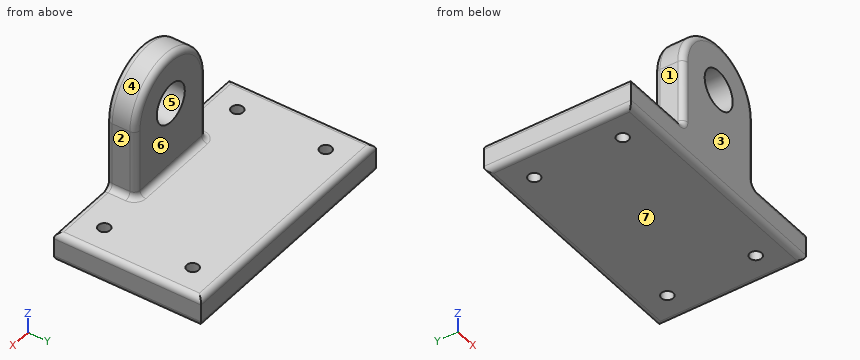
```python
from build123d import *

# Parameters (mm, degrees)
F0_W     = 125
F0_H     = 75
F1_DEPTH = 15
F2_W     = 50
F2_H     = 15
F3_DEPTH = 15
F4_R     = 3
F5_DEPTH = 15.001
F6_R     = 3


with BuildPart() as f1:
    # F0 (on Top) → F1 (new body)
    with BuildSketch(Plane.XY):
        Rectangle(F0_W, F0_H)
    extrude(amount=F1_DEPTH)

    # F2 (on face) → F3 (join)
    with BuildSketch(Plane.XZ.offset(37.5)):
        with Locations((0, 7.5)):
            Rectangle(F2_W, F2_H)
        with BuildLine():
            Line((25, 15), (25, 50))
            ThreePointArc((25, 50), (0, 25), (-25, 50))
            Line((-25, 50), (-25, 15))
            Line((-25, 15), (25, 15))
        make_face()
        with BuildLine():
            ThreePointArc((-25, 50), (0, 25), (25, 50))
            Line((25, 50), (10, 50))
            ThreePointArc((10, 50), (0, 40), (-10, 50))
            Line((-10, 50), (-25, 50))
        make_face()
        with BuildLine():
            Line((10, 50), (25, 50))
            ThreePointArc((25, 50), (0, 75), (-25, 50))
            Line((-25, 50), (-10, 50))
            ThreePointArc((-10, 50), (0, 60), (10, 50))
        make_face()
    extrude(amount=-F3_DEPTH)

    # F4 (on face) → F5 (cut, through all)
    with BuildSketch(Plane.XY.offset(15)):
        with Locations((-47.5, 22.5)):
            Circle(F4_R)
        with Locations((-47.5, -22.5)):
            Circle(F4_R)
        with Locations((47.5, 22.5)):
            Circle(F4_R)
        with Locations((47.5, -22.5)):
            Circle(F4_R)
    extrude(amount=-F5_DEPTH, mode=Mode.SUBTRACT)

    # F6
    f6_edges = [f1.edges().sort_by_distance(p)[0] for p in [
        (-43.75, -37.5, 15),
        (-62.5, 0, 15),
        (0, 37.5, 15),
        (62.5, 0, 15),
        (43.75, -37.5, 15),
        (25, -30, 15),
        (-25, -30, 15),
        (-25, -22.5, 32.5),
        (0, -37.5, 0),
        (62.5, 0, 0),
        (0, 37.5, 0),
        (-62.5, 0, 0),
        (-25, -37.5, 32.5),
        (0, -37.5, 75),
        (25, -37.5, 32.5),
        (0, -22.5, 15),
        (0, -22.5, 75),
        (25, -22.5, 32.5),
    ]]
    fillet(f6_edges, radius=F6_R)


solid = f1.part
```
Check sheet for the modelled part. Datum: model origin and axes. Units: mm. Face numbers are marked on the shaded views. A direction names the side the tool comes from. Give positions to 0.01 mm unless a question says otherwise; leave off trailing zeros. Order: outer loops, then holes, each group sorted by start corner. A loop starts at its lowest first (then second) coordinate and runs counter-clockwise, first axis right, second up. Notation, with made-up numbers: (0.25, 14.25) -> (55.25, 14.25) arc R18 ccw to (55.25, 48.25) -> close; hole circle Ø8 at (-14.5, 18.5). An arc over 180 degrees is marked (long way). Return JSON: item names as keys, results as strings.
1. Cross-section at C-C, the plane y = 22.5. Record the cut outline in (x, z), plus the area to 3 significant figures.
From the geometry:
{"outline": "(-62.5, 3) arc R3 ccw to (-59.5, 0) -> (-50.5, 0) -> (-50.5, 15) -> (-59.5, 15) arc R3 ccw to (-62.5, 12) -> close; (-44.5, 0) -> (44.5, 0) -> (44.5, 15) -> (-44.5, 15) -> close; (50.5, 0) -> (59.5, 0) arc R3 ccw to (62.5, 3) -> (62.5, 12) arc R3 ccw to (59.5, 15) -> (50.5, 15) -> close", "area": "1,690 mm^2"}
2. Set-up check for the marked faces 1, 2 and 3: record each of +Z, -Z, +X, -X, +Y, -Y from which the full face is reachable in a straight line by a thin tool's end or side.
From the geometry:
{"face 1": "+Z, -X, +Y, -Y", "face 2": "+Z, +X, +Y, -Y", "face 3": "+Z, -Z, +X, -X, -Y"}
3. Material ranges on probe 1 along Y at (x, z) = (-47.5, 4.5); probe 2 along Z at (x, y) = (0, -28); probe 3 along Z at (x, y) = (-33.5, 4.5), recorded low to high. Write a range as [from, to].
From the geometry:
{"probe 1": "[-37.5, -25.5], [-19.5, 19.5], [25.5, 37.5]", "probe 2": "[0, 40], [60, 75]", "probe 3": "[0, 15]"}
4. Go/stop test with flat-tipped pins: P1, Ø5, axis at x = 47.5, y = -22.5, coming from the +Z side; P2, Ø4.5, axis at y = -28.5, z = 42, coming from the +X side; P3, Ø9.5, axis at x = -47.5, y = 22.5, coming from the +Z side; P4, Ø1, axis at x = 3, z = 29.5, coming from the +Y side. Record where each tip stops, or that it passes through.
From the geometry:
{"P1": "through", "P2": "x = 25", "P3": "z = 15", "P4": "y = -22.5"}
5. Cross-section at B-B, the plane x = 0. Record the cut outline in (y, z).
From the geometry:
{"outline": "(-37.5, 3) arc R3 ccw to (-34.5, 0) -> (34.5, 0) arc R3 ccw to (37.5, 3) -> (37.5, 12) arc R3 ccw to (34.5, 15) -> (-19.5, 15) arc R3 cw to (-22.5, 18) -> (-22.5, 40) -> (-37.5, 40) -> close; (-37.5, 60) -> (-22.5, 60) -> (-22.5, 72) arc R3 ccw to (-25.5, 75) -> (-34.5, 75) arc R3 ccw to (-37.5, 72) -> close"}
6. Mould release check, pull along Z, two halves, no side actions. Record for the marked faces 4, 5, 6 and 7: +Z half, -Z half, draft (parallel to the pull), parting line (faces both ways), or undercut.
From the geometry:
{"face 4": "+Z half", "face 5": "undercut", "face 6": "draft", "face 7": "-Z half"}
7. Cross-section at A-A, the plane x = 47.5. Record the cut outline in (y, z), plus the area to 3 significant figures.
From the geometry:
{"outline": "(-37.5, 3) arc R3 ccw to (-34.5, 0) -> (-25.5, 0) -> (-25.5, 15) -> (-34.5, 15) arc R3 ccw to (-37.5, 12) -> close; (-19.5, 0) -> (19.5, 0) -> (19.5, 15) -> (-19.5, 15) -> close; (25.5, 0) -> (34.5, 0) arc R3 ccw to (37.5, 3) -> (37.5, 12) arc R3 ccw to (34.5, 15) -> (25.5, 15) -> close", "area": "937 mm^2"}
8. Cross-section at D-D, the plane z = 23.5. Record the cut outline in (x, y), plus the area to 3 significant figures.
From the geometry:
{"outline": "(-25, -34.5) arc R3 ccw to (-22, -37.5) -> (22, -37.5) arc R3 ccw to (25, -34.5) -> (25, -25.5) arc R3 ccw to (22, -22.5) -> (-22, -22.5) arc R3 ccw to (-25, -25.5) -> close", "area": "742 mm^2"}
